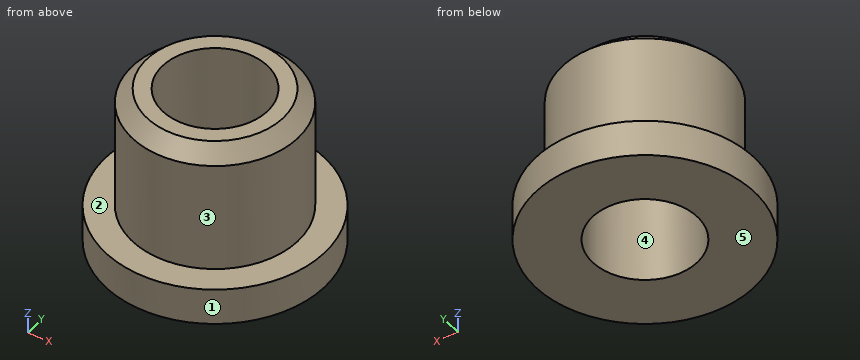
```python
from build123d import *

# Parameters (mm, degrees)
F0_R     = 5.95
F1_DEPTH = 2
F2_R     = 4.5
F3_DEPTH = 6.8
F4_R     = 2.85
F5_DEPTH = 8.801
F6_SIZE  = 0.8


with BuildPart() as f1:
    # F0 (on Top) → F1 (new body)
    with BuildSketch(Plane.XY):
        Circle(F0_R)
    extrude(amount=F1_DEPTH)

    # F2 (on face) → F3 (join)
    with BuildSketch(Plane.XY.offset(2)):
        Circle(F2_R)
    extrude(amount=F3_DEPTH)

    # F4 (on face) → F5 (cut, through all)
    with BuildSketch(Plane.XY.offset(8.8)):
        Circle(F4_R)
    extrude(amount=-F5_DEPTH, mode=Mode.SUBTRACT)

    # F6
    f6_edges = [f1.edges().sort_by_distance(p)[0] for p in [
        (-4.5, 0, 8.8),
    ]]
    chamfer(f6_edges, length=F6_SIZE)


solid = f1.part
```
Geometry check sheet. Reference: the model listing, model coordinates, mm. Face numbers are marked on the shaded views. A direction names the side the tool comes from. Give positions to 0.01 mm unless a question says otherwise; leave off trailing zeros. Write each loop counter-clockwise with the first axis right and the second up, starting at its lowest first coordinate (ties: lowest second). Pieces come first, ordered by that corner, then holes. Notation, with made-up numbers: (85, 61) -> (121, 61) arc R23 cw to (121, 70) -> close; hole circle Ø2 at (-39, -37.5). An arc over 180 degrees is marked (long way). Use one line per item in the form item = value.
Item 1: Mould release check, pull along Y, two halves, no side actions. Record for the marked faces 3, 4 and 5: released by +Y, released by -Y, zero draft, split by the parting line, or undercut.
Results list:
face_3 = split by the parting line
face_4 = undercut
face_5 = zero draft
Item 2: Sectioned sample at A-A on y = 0. Enter the section's corners in (x, z), plus the area to 3 significant figures.
Results list:
outline = (-5.95, 0) -> (-2.85, 0) -> (-2.85, 8.8) -> (-3.7, 8.8) -> (-4.5, 8) -> (-4.5, 2) -> (-5.95, 2) -> close; (2.85, 0) -> (5.95, 0) -> (5.95, 2) -> (4.5, 2) -> (4.5, 8) -> (3.7, 8.8) -> (2.85, 8.8) -> close
area = 34.2 mm2
Item 3: Access from +Z, -Z, +X, -X, +Y, -Y to the whole of each face (thin tool, end or side, straight path). Record for the marked faces 1 and 2.
Results list:
face_1 = +Z, -Z
face_2 = +Z
Item 4: Sectioned sample at D-D on z = 4.5. Enter the section's corners in (x, y), plus the area to 3 significant figures.
Results list:
outline = circle Ø9 at (0, 0); hole circle Ø5.7 at (0, 0)
area = 38.1 mm2
Item 5: Depth check by flat-ended pin: pin 1 Ø2 at (y, z) = (-3, 5.5) entering from +X; pin 2 Ø4 at (y, z) = (-4, 7.5) entering from -X; pin 3 Ø3 at (x, z) = (-1.5, 4.5) entering from +Y. Enter the tip coordinate at first touch or a pass-through.
Results list:
pin_1 = 4.03
pin_2 = -4.03
pin_3 = 4.5
Item 6: Scan lines: line 1 (Y direction, x = 0, z = 3.5); line 2 (Y direction, x = 1.25, z = 4); line 3 (X direction, y = -2, z = 0.5). Record each from-to range of solid material in increasing order.
Results list:
line_1 = -4.5 to -2.85, 2.85 to 4.5
line_2 = -4.32 to -2.56, 2.56 to 4.32
line_3 = -5.6 to -2.03, 2.03 to 5.6
Item 7: Sectioned sample at C-C on z = 1.5. Enter the section's corners in (x, y), plus the area to 3 significant figures.
Results list:
outline = circle Ø11.9 at (0, 0); hole circle Ø5.7 at (0, 0)
area = 85.7 mm2
